from build123d import *

# Parameters (mm, degrees)
F0_W     = 96.15881
F0_H     = 124.052196
F0_W_2   = 84.728866
F0_H_2   = 113.717616
F1_DEPTH = 76.2
F2_R     = 9.848118
F3_DEPTH = 127
F4_W     = 56.765504
F4_H     = 23.716378
F5_DEPTH = 127


with BuildPart() as f1:
    # F0 (on Top) → F1 (new body)
    with BuildSketch(Plane.XY):
        Rectangle(F0_W, F0_H)
        Rectangle(F0_W_2, F0_H_2, mode=Mode.SUBTRACT)
    extrude(amount=F1_DEPTH)

    # F2 (on face) → F3 (cut)
    with BuildSketch(Plane.XZ.offset(62.026098)):
        with Locations((0, 39.847784)):
            Circle(F2_R)
    extrude(amount=-F3_DEPTH, mode=Mode.SUBTRACT)

    # F4 (on face) → F5 (cut)
    with BuildSketch(Plane.YZ.offset(48.079405)):
        with Locations((0.367016, 64.341811)):
            Rectangle(F4_W, F4_H)
    extrude(amount=-F5_DEPTH, mode=Mode.SUBTRACT)


solid = f1.part
Geometry: final body of the model. Coordinates: model frame, mm. A direction names the side the tool comes from. Give positions to 0.01 mm unless a question says otherwise; leave off trailing zeros. Loops run counter-clockwise (first coordinate to the right, second up) from the corner with the lowest first, then second, coordinate; pieces in that order, holes last. Notation, with made-up numbers: M 85.5,-30 L 120.5,-30 A30 ccw 120.5,7 Z; hole C 23,-25 d1. An arc over 180 degrees is marked long. Put each result on its own line as item: value.
1) Reachability of faces 1 (the flat face through (45, 28.75, 64)), 2 (the flat face through (-42.364, -1, 29)), 3 (the flat face through (-48.079, -1, 29)) from +Z, -Z, +X, -X, +Y, -Y: full face, straight path, thin tool, end or side. Return the list, or none.
Computed values:
face 1: +Z, +X, -X
face 2: +Z, -Z
face 3: +Z, -Z, -X, +Y, -Y
2) Cut plane C-C, the plane y = -13. Return the cut outline in (x, z).
Computed values:
outline: M -48.08,0 L -42.36,0 L -42.36,52.48 L -48.08,52.48 Z; M 42.36,0 L 48.08,0 L 48.08,52.48 L 42.36,52.48 Z
3) Material intervals for L1, parallel to Z at x = 0, y = -59.45; L2, parallel to Y at x = -22, z = 49; L3, parallel to X at y = 13, z = 19.5, sorted ascending. Write a range as from..to.
Computed values:
L1: z = 0..30, 49.7..76.2
L2: y = -62.03..-56.86, 56.86..62.03
L3: x = -48.08..-42.36, 42.36..48.08
4) Cut plane A-A, the plane x = -35. Return the cut outline in (y, z).
Computed values:
outline: M -62.03,0 L -56.86,0 L -56.86,76.2 L -62.03,76.2 Z; M 56.86,0 L 62.03,0 L 62.03,76.2 L 56.86,76.2 Z
5) Mould query, pull axis Z, two halves, no side actions, for faces 4 (the flat face through (-1, -62.026, 29)), 5 (the flat face through (3, -58, 76.2)), 6 (the cylindrical face through (-2.135, 59.406, 30.234)). Classes: released by +Z, released by -Z, zero draft, split by the parting line, or undercut.
Computed values:
face 4: zero draft
face 5: released by +Z
face 6: undercut
6) Cut plane D-D, the plane z = 55. Return the cut outline in (x, y).
Computed values:
outline: M -48.08,-62.03 L 48.08,-62.03 L 48.08,-28.02 L 42.36,-28.02 L 42.36,-56.86 L -42.36,-56.86 L -42.36,-28.02 L -48.08,-28.02 Z; M -48.08,28.75 L -42.36,28.75 L -42.36,56.86 L 42.36,56.86 L 42.36,28.75 L 48.08,28.75 L 48.08,62.03 L -48.08,62.03 Z
7) Cut plane B-B, the plane x = 0. Return the cut outline in (y, z), plus the area to 3 significant figures.
Computed values:
outline: M -62.03,0 L -56.86,0 L -56.86,30 L -62.03,30 Z; M -62.03,49.7 L -56.86,49.7 L -56.86,76.2 L -62.03,76.2 Z; M 56.86,0 L 62.03,0 L 62.03,30 L 56.86,30 Z; M 56.86,49.7 L 62.03,49.7 L 62.03,76.2 L 56.86,76.2 Z
area: 584 mm^2
8) First-contact query: P1, Ø6.5, axis at x = 45.5, y = 5, coming from the +Z side; P2, Ø17.5, axis at x = 0, z = 39.85, coming from the +Y side. Flat tips, straight axial feed; report the tip coordinate or a pass-through.
Computed values:
P1: stops at z = 52.48
P2: passes through
